Source: CAD feature listing. Evaluate the final solid. Frame: model axes, mm. A direction names the side the tool comes from. Round coordinates to 2 decimals unless told otherwise and drop trailing zeros. Order: outer loops, then holes, each group sorted by start corner. A loop starts at its lowest first (then second) coordinate and runs counter-clockwise, first axis right, second up. Notation, with made-up numbers: (39.5, -29.5) -> (43.5, -29.5) arc R32 cw to (43.5, -2.5) -> close; hole circle Ø9 at (-22, 17). An arc over 180 degrees is marked (long way). Write item = value, one per line. Start each with the question number.
(1) Ray query, line 1 (X direction, y = 9, z = -7.5); line 2 (X direction, y = 21, z = -13); line 3 (Y direction, x = 19, z = -24.5). Return the intervals inside material, ascending.
(2) Cut plane B-B on y = 2. Return the cut outline in (x, z).
(3) Reachability of faces 4 (the face through (31, 28.574, -6)), 5 (the face through (30.58, 12.19, -24.98)), 6 (the face through (3.93, 29.85, -29.15)) from +Z, -Z, +X, -X, +Y, -Y: full face, straight path, thin tool, end or side. Return the list, or none.
(4) Cut plane C-C on y = 24.5. Give the number of separate pieces and of enclosed holes in the cut face, then the cut area to 3 significant figures.
(5) Cut plane A-A on x = 30. Return the cut outline in (y, z).
(6) Contact query for flat-ended pins moving along their axis: pin 1 Ø2 at (x, y) = (1.5, 22) entering from -Z; pin 2 Ø8 at (x, y) = (7, 9) entering from +Z; pin 3 Ø6 at (x, z) = (7.5, -11) entering from -Y; pin 4 Ø6 at (x, y) = (14.5, 13) entering from +Z. Output: stop coordinate, or through.
(7) Draft query along X for faces 1 (the face through (30.581, 21.416, -1.683)), 2 (the face through (32, 16, -15)), 3 (the face through (3.424, 29.851, -14.056)). Return one class per face: released by +X, released by -X, zero draft, split by the parting line, or undercut.
from build123d import *

# Parameters (mm, degrees)
SKETCH3_W               = 26.402815354
SKETCH3_H               = 30.166458461
CUT_EXTRUDE1_DEPTH      = 47
SKETCH4_R               = 1
CUT_EXTRUDE3_DEPTH      = 47
MIRROR4_COPY_1_SKETCH_R = 1
MIRROR4_COPY_1_DEPTH    = 47


with BuildPart() as part:
    # Sketch2 → Loft1 section 0
    with BuildSketch(Plane(origin=(32, 0, 0), x_dir=(0, 0, -1), z_dir=(1, 0, 0))):
        with BuildLine():
            Line((0, 14.455895325), (3.413030344, 28.573993623))
            Line((3.413030344, 28.573993623), (8.608910386, 28.573993623))
            Line((8.608910386, 28.573993623), (10.498321311, 31.093208189))
            Line((10.498321311, 31.093208189), (33.171252407, 31.093208189))
            Line((33.171252407, 31.093208189), (34.850728784, 29.833600906))
            Line((34.850728784, 29.833600906), (34.850728784, 28.573993623))
            Line((34.850728784, 28.573993623), (28.015283486, 28.573993623))
            Line((28.015283486, 28.573993623), (28.015283486, 19.565154633))
            Line((28.015283486, 19.565154633), (25.347572315, 17.820529869))
            Line((25.347572315, 17.820529869), (24.366204042, 13.129607698))
            Line((24.366204042, 13.129607698), (25.607594247, 11.231394061))
            Line((25.607594247, 11.231394061), (25.263551475, 9.586875986))
            Line((25.263551475, 9.586875986), (26.31991204, 8.508154932))
            Line((26.31991204, 8.508154932), (25.435572861, 5.355231962))
            Line((25.435572861, 5.355231962), (16.552703214, 0))
            Line((16.552703214, 0), (6.661783172, 2.774228292))
            Line((6.661783172, 2.774228292), (0, 14.455895325))
        make_face()
    # Sketch1 → Loft1 section 1
    with BuildSketch(Plane(origin=(0, 0, 0), x_dir=(0, 0, -1), z_dir=(1, 0, 0))):
        with BuildLine():
            Line((0, 14.455895325), (3.413030344, 28.573993623))
            Line((3.413030344, 28.573993623), (8.608910386, 28.573993623))
            Line((8.608910386, 28.573993623), (10.498321311, 31.093208189))
            Line((10.498321311, 31.093208189), (33.171252407, 31.093208189))
            Line((33.171252407, 31.093208189), (34.850728784, 29.833600906))
            Line((34.850728784, 29.833600906), (34.850728784, 28.573993623))
            Line((34.850728784, 28.573993623), (28.015283486, 28.573993623))
            Line((28.015283486, 28.573993623), (28.015283486, 19.565154633))
            Line((28.015283486, 19.565154633), (25.347572315, 17.820529869))
            Line((25.347572315, 17.820529869), (24.366204042, 13.129607698))
            Line((24.366204042, 13.129607698), (25.607594247, 11.231394061))
            Line((25.607594247, 11.231394061), (25.263551475, 9.586875986))
            Line((25.263551475, 9.586875986), (26.31991204, 8.508154932))
            Line((26.31991204, 8.508154932), (25.435572861, 5.355231962))
            Line((25.435572861, 5.355231962), (16.552703214, 0))
            Line((16.552703214, 0), (6.661783172, 2.774228292))
            Line((6.661783172, 2.774228292), (0, 14.455895325))
        make_face()
    loft()

    # Sketch3 → Cut-Extrude1 (cut)
    with BuildSketch(Plane.XY):
        with Locations((16, 13.490764393)):
            Rectangle(SKETCH3_W, SKETCH3_H)
    extrude(amount=-CUT_EXTRUDE1_DEPTH, mode=Mode.SUBTRACT)

    # Sketch4 → Cut-Extrude3 (cut)
    with BuildSketch(Plane(origin=(0, 31.093208189, 0), x_dir=(1, 0, 0), z_dir=(0, 1, 0))):
        with Locations(Location((4.311005364, 30.074777425, 0), (0, 0, 270))):
            Circle(SKETCH4_R)
    cut_extrude3 = extrude(amount=-CUT_EXTRUDE3_DEPTH, mode=Mode.SUBTRACT)

    # Mirror3: Cut-Extrude3 across plane
    add(cut_extrude3.mirror(Plane(origin=(16, 0, 0), x_dir=(0, 0, 1), z_dir=(1, 0, 0))), mode=Mode.SUBTRACT)

    # Mirror4: Cut-Extrude3 across plane
    add(cut_extrude3.mirror(Plane.XY.offset(-21.834786859)), mode=Mode.SUBTRACT)

    # Mirror4 copy 1 sketch → Mirror4 copy 1 (cut)
    with BuildSketch(Plane(origin=(32, 31.093208189, -43.669573718), x_dir=(-1, 0, 0), z_dir=(0, 1, 0))):
        with Locations(Location((4.311005364, 30.074777425, 0), (0, 0, 270))):
            Circle(MIRROR4_COPY_1_SKETCH_R)
    extrude(amount=-MIRROR4_COPY_1_DEPTH, mode=Mode.SUBTRACT)

    # Sketch6 → Loft2 section 0
    with BuildSketch(Plane(origin=(0, 14.288993623, 0), x_dir=(-1, 0, 0), z_dir=(0, -1, 0))):
        with BuildLine():
            Line((-9.018092228, 19.761600579), (-7.95240346, 20.196945779))
            ThreePointArc((-7.95240346, 20.196945779), (-16.127321048, 7.452302301), (-24.302238636, 20.196945779))
            Line((-24.302238636, 20.196945779), (-23.236549868, 19.761600579))
            ThreePointArc((-23.236549868, 19.761600579), (-16.127321048, 9.032071449), (-9.018092228, 19.761600579))
        make_face()
    # Sketch5 → Loft2 section 1
    with BuildSketch(Plane(origin=(0, 28.573993623, 0), x_dir=(-1, 0, 0), z_dir=(0, -1, 0))):
        with BuildLine():
            Line((-9.018092228, 24.112821073), (-7.95240346, 24.548166273))
            ThreePointArc((-7.95240346, 24.548166273), (-16.127321048, 11.803522795), (-24.302238636, 24.548166273))
            Line((-24.302238636, 24.548166273), (-23.236549868, 24.112821073))
            ThreePointArc((-23.236549868, 24.112821073), (-16.127321048, 13.383291944), (-9.018092228, 24.112821073))
        make_face()
    loft()


solid = part.part
Evaluation:
q1.line_1 = 0 to 2.8, 29.2 to 32
q1.line_2 = 0 to 2.8, 9 to 11.03, 21.23 to 23.25, 29.2 to 32
q1.line_3 = 28.57 to 31.09
q2.outline = (0, -19.87) -> (2.8, -19.87) -> (2.8, -9.42) -> (0, -9.42) -> close; (29.2, -19.87) -> (32, -19.87) -> (32, -9.42) -> (29.2, -9.42) -> close
q3.face_4 = +Z, +X, -X, +Y
q3.face_5 = -Z, +X, -X
q3.face_6 = +Y, -Y
q4.separate_pieces = 3
q4.enclosed_holes = 0
q4.area = 190 mm^2
q5.outline = (0, -16.55) -> (5.36, -25.44) -> (8.51, -26.32) -> (9.59, -25.26) -> (11.23, -25.61) -> (13.13, -24.37) -> (17.82, -25.35) -> (19.57, -28.02) -> (28.57, -28.02) -> (28.57, -34.85) -> (29.83, -34.85) -> (31.09, -33.17) -> (31.09, -10.5) -> (28.57, -8.61) -> (28.57, -3.41) -> (14.46, 0) -> (2.77, -6.66) -> close
q6.pin_1 = -28.02
q6.pin_2 = through
q6.pin_3 = 14.29
q6.pin_4 = -7.45
q7.face_1 = zero draft
q7.face_2 = released by +X
q7.face_3 = undercut
